Input: part model. Units: mm. Frame: model coordinates. A direction names the side the tool comes from. Give positions to 0.01 mm unless a question says otherwise; leave off trailing zeros. Order: outer loops, then holes, each group sorted by start corner. A loop starts at its lowest first (then second) coordinate and runs counter-clockwise, first axis right, second up.
```python
from build123d import *

# Parameters (mm, degrees)
SKETCH1_W                         = 100
SKETCH1_H                         = 70
BASE_FLANGE1_DEPTH                = 3
EDGE_FLANGE1_STRIP_W              = 12.3
EDGE_FLANGE1_STRIP_H              = 3
EDGE_FLANGE1_STRIP_CUT_DEPTH      = 70
EDGE_FLANGE1_DEPTH                = 70
EDGE_FLANGE3_STRIP_W              = 12.3
EDGE_FLANGE3_STRIP_H              = 3
EDGE_FLANGE3_STRIP_CUT_DEPTH      = 70
EDGE_FLANGE3_DEPTH                = 70
TAP_START                         = -47
TAP_DRILL_SLOT_FOR_M5_TAP3_DEPTH  = 48
TAP_DRILL_FOR_M5_TAP1_D           = 4.2
TAP_DRILL_FOR_M5_TAP1_CSINK_D     = 4.25
TAP_DRILL_FOR_M5_TAP1_CSINK_ANGLE = 90


with BuildPart() as part:
    # Base-Flange1: sheet metal written as solids
    # Sketch1 → Base-Flange1 (new body)
    with BuildSketch(Plane.XY):
        with Locations((9.007487246, 428.98845549)):
            Rectangle(SKETCH1_W, SKETCH1_H)
    extrude(amount=-BASE_FLANGE1_DEPTH)

    # Edge-Flange1: sheet metal written as solids
    # Edge-Flange1 strip (on a plane across the edge) → Edge-Flange1 strip cut (cut)
    with BuildSketch(Plane(origin=(-40.992512754, 393.98845549, -3), x_dir=(1, 0, 0), z_dir=(0, 1, 0))):
        with Locations((-6, -1.5)):
            Rectangle(EDGE_FLANGE1_STRIP_W, EDGE_FLANGE1_STRIP_H)
    extrude(amount=EDGE_FLANGE1_STRIP_CUT_DEPTH, mode=Mode.SUBTRACT)

    # Edge-Flange1 section (on a plane across the edge) → Edge-Flange1 (add)
    with BuildSketch(Plane(origin=(-40.992512754, 393.98845549, -3), x_dir=(1, 0, 0), z_dir=(0, 1, 0))):
        with BuildLine():
            Line((-3, 0.15), (-3, 40))
            Line((-3, 40), (0, 40))
            Line((0, 40), (0, 0.15))
            ThreePointArc((0, 0.15), (0.043933983, 0.043933983), (0.15, 0))
            Line((0.15, 0), (0.15, -3))
            ThreePointArc((0.15, -3), (-2.077386361, -2.077386361), (-3, 0.15))
        make_face()
    extrude(amount=EDGE_FLANGE1_DEPTH)

    # Edge-Flange3: sheet metal written as solids
    # Edge-Flange3 strip (on a plane across the edge) → Edge-Flange3 strip cut (cut)
    with BuildSketch(Plane(origin=(-40.992512754, 393.98845549, -43), x_dir=(0, 0, 1), z_dir=(0, 1, 0))):
        with Locations((-6, -1.5)):
            Rectangle(EDGE_FLANGE3_STRIP_W, EDGE_FLANGE3_STRIP_H)
    extrude(amount=EDGE_FLANGE3_STRIP_CUT_DEPTH, mode=Mode.SUBTRACT)

    # Edge-Flange3 section (on a plane across the edge) → Edge-Flange3 (add)
    with BuildSketch(Plane(origin=(-40.992512754, 393.98845549, -43), x_dir=(0, 0, 1), z_dir=(0, 1, 0))):
        with BuildLine():
            Line((-3, 0.15), (-3, 100))
            Line((-3, 100), (0, 100))
            Line((0, 100), (0, 0.15))
            ThreePointArc((0, 0.15), (0.043933983, 0.043933983), (0.15, 0))
            Line((0.15, 0), (0.15, -3))
            ThreePointArc((0.15, -3), (-2.077386361, -2.077386361), (-3, 0.15))
        make_face()
    extrude(amount=EDGE_FLANGE3_DEPTH)

    # Tap Drill Slot for M5 Tap3: read off the stored shape, not the designer's step
    # Tap Drill Slot for M5 Tap3 outline → Tap Drill Slot for M5 Tap3 (cut)
    with BuildSketch(Plane.XY.offset(TAP_START)):
        with BuildLine():
            ThreePointArc((12.657487246, 431.08845549), (10.557487246, 428.98845549), (12.657487246, 426.88845549))
            Line((12.657487246, 426.88845549), (25.357487246, 426.88845549))
            ThreePointArc((25.357487246, 426.88845549), (27.457487246, 428.98845549), (25.357487246, 431.08845549))
            Line((25.357487246, 431.08845549), (12.657487246, 431.08845549))
        make_face()
        with BuildLine():
            ThreePointArc((-27.342512754, 431.08845549), (-29.442512754, 428.98845549), (-27.342512754, 426.88845549))
            Line((-27.342512754, 426.88845549), (-14.642512754, 426.88845549))
            ThreePointArc((-14.642512754, 426.88845549), (-12.542512754, 428.98845549), (-14.642512754, 431.08845549))
            Line((-14.642512754, 431.08845549), (-27.342512754, 431.08845549))
        make_face()
    extrude(amount=TAP_DRILL_SLOT_FOR_M5_TAP3_DEPTH, mode=Mode.SUBTRACT)

    # Tap Drill Slot for M5 Tap3 2: loft between two sections, ruled curve by curve
    tap_drill_slot_for_m5_tap3_2_from = [
        Edge.make_three_point_arc((25.357487246, 426.88845549, -0.025), (26.842411487, 427.503531249, -0.025), (27.457487246, 428.98845549, -0.025)),
        Edge.make_three_point_arc((27.457487246, 428.98845549, -0.025), (26.842411487, 430.47337973, -0.025), (25.357487246, 431.08845549, -0.025)),
        Edge.make_three_point_arc((12.657487246, 431.08845549, -0.025), (11.172563006, 430.47337973, -0.025), (10.557487246, 428.98845549, -0.025)),
        Edge.make_three_point_arc((10.557487246, 428.98845549, -0.025), (11.172563006, 427.503531249, -0.025), (12.657487246, 426.88845549, -0.025)),
        Edge.make_line((25.357487246, 431.08845549, -0.025), (12.657487246, 431.08845549, -0.025)),
        Edge.make_line((25.357487246, 426.88845549, -0.025), (12.657487246, 426.88845549, -0.025)),
    ]
    tap_drill_slot_for_m5_tap3_2_to = [
        Edge.make_three_point_arc((25.357487246, 426.86345549, 0), (26.860089156, 427.48585358, 0), (27.482487246, 428.98845549, 0)),
        Edge.make_three_point_arc((27.482487246, 428.98845549, 0), (26.860089156, 430.4910574, 0), (25.357487246, 431.11345549, 0)),
        Edge.make_three_point_arc((12.657487246, 431.11345549, 0), (11.154885336, 430.4910574, 0), (10.532487246, 428.98845549, 0)),
        Edge.make_three_point_arc((10.532487246, 428.98845549, 0), (11.154885336, 427.48585358, 0), (12.657487246, 426.86345549, 0)),
        Edge.make_line((25.357487246, 431.11345549, 0), (12.657487246, 431.11345549, 0)),
        Edge.make_line((25.357487246, 426.86345549, 0), (12.657487246, 426.86345549, 0)),
    ]
    tap_drill_slot_for_m5_tap3_2 = Solid(Shell([*[Face.make_surface_from_curves(tap_drill_slot_for_m5_tap3_2_from[k], tap_drill_slot_for_m5_tap3_2_to[k]) for k in range(6)], Face(Wire(tap_drill_slot_for_m5_tap3_2_from)), Face(Wire(tap_drill_slot_for_m5_tap3_2_to))]))
    add(tap_drill_slot_for_m5_tap3_2, mode=Mode.SUBTRACT)

    # Tap Drill Slot for M5 Tap3 3: loft between two sections, ruled curve by curve
    tap_drill_slot_for_m5_tap3_3_from = [
        Edge.make_three_point_arc((-14.642512754, 426.88845549, -0.025), (-13.157588513, 427.503531249, -0.025), (-12.542512754, 428.98845549, -0.025)),
        Edge.make_three_point_arc((-12.542512754, 428.98845549, -0.025), (-13.157588513, 430.47337973, -0.025), (-14.642512754, 431.08845549, -0.025)),
        Edge.make_three_point_arc((-27.342512754, 431.08845549, -0.025), (-28.827436994, 430.47337973, -0.025), (-29.442512754, 428.98845549, -0.025)),
        Edge.make_three_point_arc((-29.442512754, 428.98845549, -0.025), (-28.827436994, 427.503531249, -0.025), (-27.342512754, 426.88845549, -0.025)),
        Edge.make_line((-14.642512754, 431.08845549, -0.025), (-27.342512754, 431.08845549, -0.025)),
        Edge.make_line((-14.642512754, 426.88845549, -0.025), (-27.342512754, 426.88845549, -0.025)),
    ]
    tap_drill_slot_for_m5_tap3_3_to = [
        Edge.make_three_point_arc((-14.642512754, 426.86345549, 0), (-13.139910844, 427.48585358, 0), (-12.517512754, 428.98845549, 0)),
        Edge.make_three_point_arc((-12.517512754, 428.98845549, 0), (-13.139910844, 430.4910574, 0), (-14.642512754, 431.11345549, 0)),
        Edge.make_three_point_arc((-27.342512754, 431.11345549, 0), (-28.845114664, 430.4910574, 0), (-29.467512754, 428.98845549, 0)),
        Edge.make_three_point_arc((-29.467512754, 428.98845549, 0), (-28.845114664, 427.48585358, 0), (-27.342512754, 426.86345549, 0)),
        Edge.make_line((-14.642512754, 431.11345549, 0), (-27.342512754, 431.11345549, 0)),
        Edge.make_line((-14.642512754, 426.86345549, 0), (-27.342512754, 426.86345549, 0)),
    ]
    tap_drill_slot_for_m5_tap3_3 = Solid(Shell([*[Face.make_surface_from_curves(tap_drill_slot_for_m5_tap3_3_from[k], tap_drill_slot_for_m5_tap3_3_to[k]) for k in range(6)], Face(Wire(tap_drill_slot_for_m5_tap3_3_from)), Face(Wire(tap_drill_slot_for_m5_tap3_3_to))]))
    add(tap_drill_slot_for_m5_tap3_3, mode=Mode.SUBTRACT)

    # Tap Drill for M5 Tap1 (through all)
    with Locations(Plane.ZY.offset(43.992512754)):
        with Locations((-34.85, 439.23845549), (-11.15, 439.23845549), (-11.15, 418.73845549), (-34.85, 418.73845549)):
            CounterSinkHole(TAP_DRILL_FOR_M5_TAP1_D / 2, TAP_DRILL_FOR_M5_TAP1_CSINK_D / 2, counter_sink_angle=TAP_DRILL_FOR_M5_TAP1_CSINK_ANGLE)


solid = part.part
```
1) Pull-direction query (X, two-part tool) for faces 1 (the face through (-29.442, 429.035, -1.533)), 2 (the face through (59.007, 428, -1)), 3 (the face through (-43.045, 428.498, -0.898)); classes: pulls with the +X half, pulls with the -X half, needs draft (parallel to the pull), parting line crosses it, or undercut.
2) Reachability of faces 4 (the face through (8, 429, -3)), 5 (the face through (-42.46, 437.19, -34.39)), 6 (the face through (27.457, 428.942, -44.521)) from +Z, -Z, +X, -X, +Y, -Y: full face, straight path, thin tool, end or side. Return the list, or none.
3) First-contact query: P1, Ø20, axis at y = 440.5, z = -18.5, coming from the +X side. Flat tip, straight axial feed; report the tip coordinate or a pass-through.
4) Line query: probe 1 along Y at (x, z) = (-42.05, -11.15); probe 2 along Z at (x, y) = (43, 432); probe 3 along X at (y, z) = (424, -36). Output: solid intervals per line, ascending.
5) Cut plane C-C (y = 412.5). Return the cut outline in (x, z).
6) Cut plane A-A (x = 35.5). Return the cut outline in (y, z).
7) Cut plane B-B (z = -34.85). Count the separate pieces of the cut face and the enclosed holes in it, then the cut area to 3 significant figures.
Geometry says:
1. face 1: undercut
1. face 2: pulls with the +X half
1. face 3: pulls with the -X half
2. face 4: +X, +Y, -Y
2. face 5: +X, -X
2. face 6: +Z, -Z
3. P1: stops at x = -40.99
4. probe 1: y = 393.99 to 416.64, 420.84 to 437.14, 441.34 to 463.99
4. probe 2: z = -46 to -43, -3 to 0
4. probe 3: x = -43.99 to -40.99
5. outline: (-43.99, -42.85) arc R3.15 ccw to (-40.84, -46) - (59.01, -46) - (59.01, -43) - (-40.84, -43) arc R0.15 cw to (-40.99, -42.85) - (-40.99, -3.15) arc R0.15 cw to (-40.84, -3) - (59.01, -3) - (59.01, 0) - (-40.84, 0) arc R3.15 ccw to (-43.99, -3.15) - close
6. outline: (393.99, -46) - (463.99, -46) - (463.99, -43) - (393.99, -43) - close; (393.99, -3) - (463.99, -3) - (463.99, 0) - (393.99, 0) - close
7. separate pieces: 3
7. enclosed holes: 0
7. area: 185 mm2
